Geometry: see drawing. Coordinates: mm, zero at the bounding-box minimum. Coordinates: 2 decimals unless noted, no trailing zeros. Write each loop counter-clockwise with the first axis right and the second up, starting at its lowest first coordinate (ties: lowest second). Pieces come first, ordered by that corner, then holes.
1) Section query B-B (y = 7.5). Output: boundary loops of the cut face in (x, z), then the cut area to 3 significant figures.
2) Section query A-A (y = 3). Output: boundary loops of the cut face in (x, z), then the cut area to 3 significant figures.
3) Pin query (flat end, axial travel): pin 1 Ø1.8 at (x, y) = (31, 3) entering from -Z; pin 2 Ø1.5 at (x, y) = (22, 3.5) entering from -Z. Return the tip coordinate at first contact, or that it passes through.
4) Section query C-C (x = 7.5). Output: boundary loops of the cut face in (y, z).
5) Line query: L1, parallel to Y at x = 22.5, z = 0.6; L2, parallel to Y at x = 31, z = 0.2; L3, parallel to X at y = 7.25, z = 0.85. Output: solid intervals per line, ascending.
6) Section query D-D (z = 1.15). Output: boundary loops of the cut face in (x, y), then the cut area to 3 significant figures.
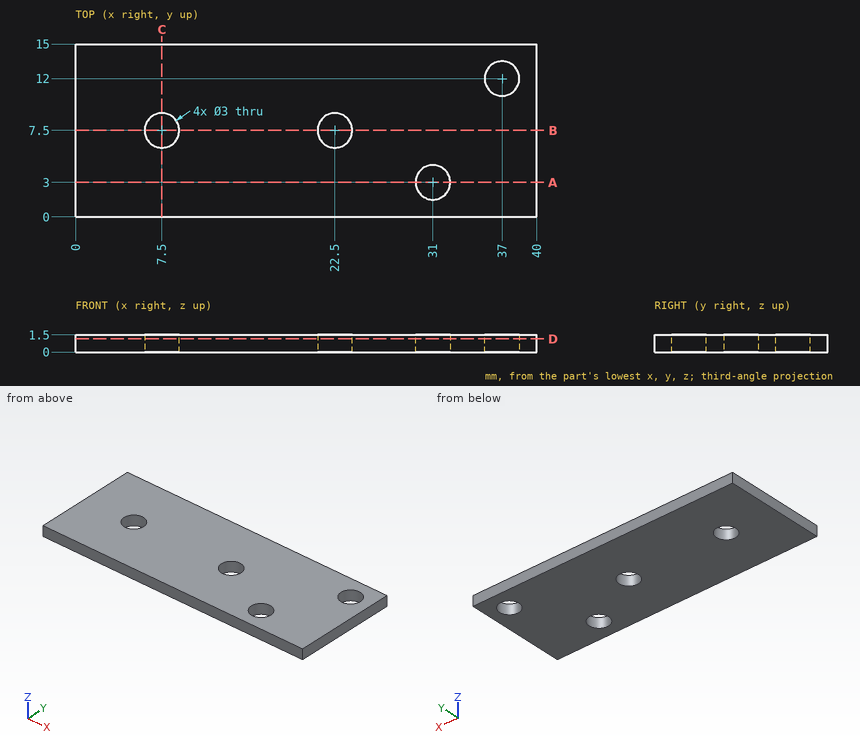
Answer:
1. outline: (0, 0) - (6, 0) - (6, 1.5) - (0, 1.5) - close; (9, 0) - (21, 0) - (21, 1.5) - (9, 1.5) - close; (24, 0) - (40, 0) - (40, 1.5) - (24, 1.5) - close
1. area: 51.0 mm2
2. outline: (0, 0) - (29.5, 0) - (29.5, 1.5) - (0, 1.5) - close; (32.5, 0) - (40, 0) - (40, 1.5) - (32.5, 1.5) - close
2. area: 55.5 mm2
3. pin 1: passes through
3. pin 2: stops at z = 0
4. outline: (0, 0) - (6, 0) - (6, 1.5) - (0, 1.5) - close; (9, 0) - (15, 0) - (15, 1.5) - (9, 1.5) - close
5. L1: y = 0 to 6, 9 to 15
5. L2: y = 0 to 1.5, 4.5 to 15
5. L3: x = 0 to 6.02, 8.98 to 21.02, 23.98 to 40
6. outline: (0, 0) - (40, 0) - (40, 15) - (0, 15) - close; hole circle Ø3 at (7.5, 7.5); hole circle Ø3 at (22.5, 7.5); hole circle Ø3 at (31, 3); hole circle Ø3 at (37, 12)
6. area: 572 mm2
